Autodesk Inventor part; units mm, degrees
ref_plane "YZ Plane" through (0, 0, 0) normal (1, 0, 0) x (0, 1, 0)
ref_plane "XZ Plane" through (0, 0, 0) normal (0, 1, 0) x (-1, 0, 0)
ref_plane "XY Plane" through (0, 0, 0) normal (0, 0, 1) x (1, 0, 0)
sketch "Skizze1" plane through (0, 0, 0) normal (0, 0, 1) x (1, 0, 0)
  line L0 (-0.8667, 0) -> (6, 0)
  line L1 (6, 0) -> (6, 1.5)
  line L2 (6, 1.5) -> (1.25, 1.5)
  line L3 (1.25, 1.5) -> (0.9432, 1.5)
  line L4 (0.9432, 1.5) -> (0, 1.5)
  line L5 (0, 1.5) -> (0, 2.75)
  line L6 (0, 2.75) -> (-3, 2.75)
  line L7 (-3, 2.75) -> (-3, 1.4434)
  line L8 (-3, 1.4434) -> (-1.7, 1.4434)
  line L9 (-1.7, 1.4434) -> (-0.8667, 0)
  line L10 (-15.5, 0) -> (61.5, 0)
  line L11 (0, -0.8) -> (0, 10.4)
  line L12 (1.25, 1.5) -> (0, 1.5) construction
  dimension "d1" = 4.75
  dimension "d2" = 0.3068
  dimension "d3" = 3
  dimension "d4" = 1.3
  dimension "d5" = 60
  dimension "d6" = 3
  dimension "d7" = 3
  dimension "d8" = 2.8868
  dimension "d9" = 5.5
  dimension "d26" = 6
revolve "Körper" add sketch "Skizze1" angle 360 about axis through (-0.8667, 0, 0) along (1, 0, 0)
sketch "Skizze2" plane through (-3, 0, 0) normal (-1, 0, 0) x (0, 0, 1)
  circle A0 centre (0, 0) radius 1.4434
  line L0 (0, -3.3) -> (0, 4.4)
  line L1 (-3.3, 0) -> (4.4, 0)
  line L2 (1.4434, 0) -> (0.7217, -1.25)
  line L3 (0.7217, -1.25) -> (-0.7217, -1.25)
  line L4 (-0.7217, -1.25) -> (-1.4434, 0)
  line L5 (-1.4434, 0) -> (-0.7217, 1.25)
  line L6 (-0.7217, 1.25) -> (0.7217, 1.25)
  line L7 (0.7217, 1.25) -> (1.4434, 0)
extrude "Loch" add sketch "Skizze2" against normal up to next contours L7 A0 | A0 L2 | L6 L0 A0 | A0 L0 L3 | L0 L6 A0 | A0 L3 L0 | L4 A0 | A0 L5
fillet "Rundung1" radius 0.3 1 edges at (-3, -2.75, 0)
thread "Gewinde"
chamfer "Fase1" distance 0.3067 distance2 0.3067 1 edges at (6, -1.5, 0) measured on face at (6, -0.2617, -0.7882)
equation "\"d1\" = GEL"
equation "\"d3\" = KOH"
equation "\"d4\" = INTI"
equation "\"d6\" = GD"
equation "\"d7\" = BDM"
equation "\"d8\" = 1.1547 * SW"
equation "\"d9\" = KOD"
equation "\"d26\" = NLG"
equation "\"d17\" = RR"
equation "\"d13\" = GEL"
equation "\"d15\" = -0.5 * SPD + 0.5 * GD"
equation "\"d16\" = GUL"
equation "\"GD\" = NND"
equation "\"NLG\" = 6"
equation "\"GEL\" = 4.75"
equation "\"KOD\" = 5.5"
equation "\"KOH\" = 3"
equation "\"INTI\" = 1.3"
equation "\"GAL\" = 0.61345 * TPU"
equation "\"GUL\" = 0.61345 * TPU"
equation "\"BDM\" = NND"
equation "\"SW\" = 2.5"
equation "\"RR\" = 0.1 * KOH"
equation "\"SPD\" = NND - 1.2269 * TPU"
equation "\"NND\" = 3"
equation "\"E0\" = 1.155 * SW"
equation "\"ANG\" = 120deg"
equation "\"FAWI\" = 45deg"
equation "\"THREADDIA\" = 3"
equation "\"TPU\" = 0.5"
equation "\"GD1\" = THREADDIA - 1.2269 * TPU"
equation "\"PTC\" = TPU"
equation "\"TOA\" = 30deg"
properties part number "520204172"
The model under review builds one solid part; all positions refer to its coordinate system, in mm. A direction names the side the tool comes from. Coordinates: 2 decimals unless noted, no trailing zeros. Order: outer loops, then holes, each group sorted by start corner. A loop starts at its lowest first (then second) coordinate and runs counter-clockwise, first axis right, second up. Notation, with made-up numbers: M -22.5,86.25 L 34.5,86.25 A17 ccw 34.5,106.25 Z; hole C 64,59 d8. An arc over 180 degrees is marked long. One line per question, with ' | ' between items.
(1) Insertion check: pin 1 (1.5 mm diameter, centred on x = 0.5, y = 0, fed in from -Z); pin 2 (1 mm diameter, centred on x = 1, z = 1.5, fed in from -Y). Each pin has a flat end and moves straight along its axis. Give the tip position at first contact, or say it passes through.
Geometry results:
pin 1: stops at z = -2.75 | pin 2: stops at y = -1.12
(2) Add section B-B, the plane x = -0.75. Write out the cut boundary in (y, z).
Geometry results:
outline: C 0,0 d5.5
(3) Machinability: for faces 4 (the face through (-3, -1.1, 1.1)), 5 (the face through (-2.304, 0.616, -1.088)), which of the approach directions +Z, -Z, +X, -X, +Y, -Y give a long, thin tool a straight path to every point of the face, cutting with its end or side? Answer none if there is none.
Geometry results:
face 4: +Z, -Z, -X, +Y, -Y | face 5: -X
(4) For probe 1 along X at (y, z) = (-0.55, -1.65); probe 2 along X at (y, z) = (0.5, 0.85); probe 3 along Y at (x, z) = (-0.75, 1.85), list the stretches that pass through material, from the lowest coordinate up. Write a range as from..to.
Geometry results:
probe 1: x = -3..0 | probe 2: x = -1.44..6 | probe 3: y = -2.03..2.03
(5) The part is to be moulded in two halves that separate along Y. For faces 1 (the face through (0, 1.2, -1.2)), 2 (the face through (2.81, -1.5, -0.07)), 3 (the face through (-2, -1.25, 0)), say which applies: +Y half, -Y half, draft (parallel to the pull), parting line (faces both ways), or undercut.
Geometry results:
face 1: draft | face 2: parting line | face 3: undercut
(6) Add section A-A, the plane x = 0.25. Write out the cut boundary in (y, z), then the cut area to 3 significant figures.
Geometry results:
outline: C 0,0 d3 | area: 7.07 mm²
